Source: CAD feature listing. Evaluate the final solid. Frame: model axes, mm. A direction names the side the tool comes from. Give positions to 0.01 mm unless a question says otherwise; leave off trailing zeros. Order: outer loops, then holes, each group sorted by start corner. A loop starts at its lowest first (then second) coordinate and runs counter-clockwise, first axis right, second up.
from build123d import *

# Parameters (mm, degrees)
SKETCH1_W                                  = 280
SKETCH1_H                                  = 150
BOSS_EXTRUDE1_DEPTH                        = 20
SKETCH2_W                                  = 30
SKETCH2_H                                  = 30
BOSS_EXTRUDE2_DEPTH                        = 20
MIRROR1_AT_THE_SECOND_PLANE_COPY_1_SKETC_W = 30
MIRROR1_AT_THE_SECOND_PLANE_COPY_1_SKETC_H = 30
MIRROR1_AT_THE_SECOND_PLANE_COPY_1_DEPTH   = 20
SKETCH3_R                                  = 2.5
BOSS_EXTRUDE3_DEPTH                        = 160
SKETCH7_W                                  = 280
SKETCH7_H                                  = 50
BOSS_EXTRUDE5_DEPTH                        = 40
SKETCH8_R                                  = 7.5
CUT_EXTRUDE1_DEPTH                         = 321.156211872


with BuildPart() as part:
    # Sketch1 → Boss-Extrude1 (new body)
    with BuildSketch(Plane(origin=(0, 0, 0), x_dir=(1, 0, 0), z_dir=(0, 1, 0))):
        with Locations((-140, 75)):
            Rectangle(SKETCH1_W, SKETCH1_H)
    extrude(amount=-BOSS_EXTRUDE1_DEPTH)

    # Sketch2 → Boss-Extrude2 (add)
    with BuildSketch(Plane.XZ.offset(20)):
        with Locations((-235, -15)):
            Rectangle(SKETCH2_W, SKETCH2_H)
    boss_extrude2 = extrude(amount=BOSS_EXTRUDE2_DEPTH)

    # Mirror1: Boss-Extrude2 across plane
    add(boss_extrude2.mirror(Plane.ZY.offset(140)))

    # Mirror1 at the second plane: Boss-Extrude2 across plane
    add(boss_extrude2.mirror(Plane(origin=(0, 0, -75), x_dir=(1, 0, 0), z_dir=(0, 0, -1))))

    # Mirror1 at the second plane copy 1 sketc → Mirror1 at the second plane copy 1 (add)
    with BuildSketch(Plane(origin=(-280, -20, -150), x_dir=(-1, 0, 0), z_dir=(0, -1, 0))):
        with Locations((-235, -15)):
            Rectangle(MIRROR1_AT_THE_SECOND_PLANE_COPY_1_SKETC_W, MIRROR1_AT_THE_SECOND_PLANE_COPY_1_SKETC_H)
    extrude(amount=MIRROR1_AT_THE_SECOND_PLANE_COPY_1_DEPTH)

    # Sketch3 → Boss-Extrude3 (add)
    with BuildSketch(Plane(origin=(-220, 0, 0), x_dir=(0, 0, -1), z_dir=(1, 0, 0))):
        with Locations(Location((7.5, -30, 0), (0, 0, 180))):
            Circle(SKETCH3_R)
        with Locations(Location((22.5, -30, 0), (0, 0, 180))):
            Circle(SKETCH3_R)
    boss_extrude3 = extrude(amount=BOSS_EXTRUDE3_DEPTH)

    # Mirror2: Boss-Extrude3 across plane
    add(boss_extrude3.mirror(Plane(origin=(0, 0, -75), x_dir=(1, 0, 0), z_dir=(0, 0, -1))))

    # Sketch7 → Boss-Extrude5 (add)
    with BuildSketch(Plane(origin=(0, 0, 0), x_dir=(1, 0, 0), z_dir=(0, 1, 0))):
        with Locations((-140, 125)):
            Rectangle(SKETCH7_W, SKETCH7_H)
    boss_extrude5 = extrude(amount=BOSS_EXTRUDE5_DEPTH)

    # Mirror4: Boss-Extrude5 across plane
    add(boss_extrude5.mirror(Plane(origin=(0, 0, -75), x_dir=(1, 0, 0), z_dir=(0, 0, -1))))

    # Sketch8 → Cut-Extrude1 (cut, through all)
    with BuildSketch(Plane(origin=(0, 0, -150), x_dir=(-1, 0, 0), z_dir=(0, 0, -1))):
        with Locations((25, 20)):
            Circle(SKETCH8_R)
        with Locations((65, 20)):
            Circle(SKETCH8_R)
        with Locations((215, 20)):
            Circle(SKETCH8_R)
        with Locations((255, 20)):
            Circle(SKETCH8_R)
    extrude(amount=-CUT_EXTRUDE1_DEPTH, mode=Mode.SUBTRACT)


solid = part.part
1) Pull-direction query (Z, two-part tool) for faces 6 (the face through (-142, 8, 0)), 7 (the face through (-222.154, 22.253, -125.35)), 8 (the face through (-235, -30, -120)); classes: +Z half, -Z half, draft (parallel to the pull), parting line (faces both ways), or undercut.
Checks:
face 6: +Z half
face 7: draft
face 8: undercut
2) Section query A-A on x = -210.5. Output: boundary loops of the cut face in (y, z), and give its area (3 significant figures).
Checks:
outline: circle Ø5 at (-30, -142.5); circle Ø5 at (-30, -127.5); circle Ø5 at (-30, -22.5); circle Ø5 at (-30, -7.5); (-20, -150) - (14, -150) - (14, -100) - (0, -100) - (0, -50) - (14, -50) - (14, 0) - (-20, 0) - close; (26, -150) - (40, -150) - (40, -100) - (26, -100) - close; (26, -50) - (40, -50) - (40, 0) - (26, 0) - close
area: 5,880 mm2
3) Section query D-D on x = -25. Output: boundary loops of the cut face in (y, z), and give its area (3 significant figures).
Checks:
outline: (-20, -150) - (12.5, -150) - (12.5, -100) - (0, -100) - (0, -50) - (12.5, -50) - (12.5, 0) - (-20, 0) - close; (27.5, -150) - (40, -150) - (40, -100) - (27.5, -100) - close; (27.5, -50) - (40, -50) - (40, 0) - (27.5, 0) - close
area: 5,500 mm2
4) First-contact query: pin 1 Ø4 at (x, z) = (-44.5, -54.5) entering from +Y; pin 2 Ø10 at (y, z) = (-33, -129.5) entering from +X; pin 3 Ø2 at (x, y) = (-199.5, -27.5) entering from -Z; pin 4 Ø13.5 at (x, y) = (-65, 20) entering from -Z. Flat tips, straight axial feed; report the tip coordinate or a pass-through.
Checks:
pin 1: stops at y = 0
pin 2: stops at x = -30
pin 3: stops at z = -144.5
pin 4: passes through
5) Reachability of faces 1 (the face through (-250, -30, -15)), 2 (the face through (-30, -30, -15)), 3 (the face through (-142, 20, -100)), 4 (the face through (-45, -30, -30)), 5 (the face through (-220, -30, -15)) from +Z, -Z, +X, -X, +Y, -Y: full face, straight path, thin tool, end or side. Return the list, or none.
Checks:
face 1: +Z, -Z, -X, -Y
face 2: +Z, -Z, +X, -Y
face 3: +X, -X, +Y
face 4: +X, -X, -Y
face 5: none
6) Section query B-B on z = -113.5. Output: boundary loops of the cut face in (x, y).
Checks:
outline: (-280, -20) - (0, -20) - (0, 40) - (-280, 40) - close; hole circle Ø15 at (-255, 20); hole circle Ø15 at (-215, 20); hole circle Ø15 at (-65, 20); hole circle Ø15 at (-25, 20)
7) Ray query, L1, parallel to Y at x = -65, z = -36; L2, parallel to Z at x = -259, y = 36.5; L3, parallel to Y at x = -227.5, z = -94. Return the intervals inside material, ascending.
Checks:
L1: y = -20 to 12.5, 27.5 to 40
L2: z = -150 to -100, -50 to 0
L3: y = -20 to 0
8) Section query C-C on y = 9.5. Output: boundary loops of the cut face in (x, z), and give its area (3 significant figures).
Checks:
outline: (-280, -150) - (0, -150) - (0, -100) - (-280, -100) - close; (-280, -50) - (0, -50) - (0, 0) - (-280, 0) - close
area: 28,000 mm2
